from build123d import *

# Parameters (mm, degrees)
SKETCH1_R           = 2.1
BOSS_EXTRUDE1_DEPTH = 20
SKETCH2_W           = 74
SKETCH2_H           = 111
CUT_EXTRUDE1_DEPTH  = 18


with BuildPart() as part:
    # Sketch1 → Boss-Extrude1 (new body)
    with BuildSketch(Plane(origin=(0, 0, 0), x_dir=(1, 0, 0), z_dir=(0, 1, 0))):
        with BuildLine():
            Line((-55.8, 60), (55.8, 60))
            ThreePointArc((55.8, 60), (58.769848481, 58.769848481), (60, 55.8))
            Line((60, 55.8), (60, -55.8))
            ThreePointArc((60, -55.8), (58.769848481, -58.769848481), (55.8, -60))
            Line((55.8, -60), (-55.8, -60))
            ThreePointArc((-55.8, -60), (-58.769848481, -58.769848481), (-60, -55.8))
            Line((-60, -55.8), (-60, 55.8))
            ThreePointArc((-60, 55.8), (-58.769848481, 58.769848481), (-55.8, 60))
        make_face()
        with Locations(Location((50, 50, 0), (0, 0, 270))):
            Circle(SKETCH1_R, mode=Mode.SUBTRACT)
        with Locations(Location((-50, 50, 0), (0, 0, 90))):
            Circle(SKETCH1_R, mode=Mode.SUBTRACT)
        with Locations(Location((50, -50, 0), (0, 0, 90))):
            Circle(SKETCH1_R, mode=Mode.SUBTRACT)
        with Locations(Location((-50, -50, 0), (0, 0, 270))):
            Circle(SKETCH1_R, mode=Mode.SUBTRACT)
    extrude(amount=BOSS_EXTRUDE1_DEPTH)

    # Sketch2 → Cut-Extrude1 (cut)
    with BuildSketch(Plane(origin=(0, 20, 0), x_dir=(1, 0, 0), z_dir=(0, 1, 0))):
        Rectangle(SKETCH2_W, SKETCH2_H)
    extrude(amount=-CUT_EXTRUDE1_DEPTH, mode=Mode.SUBTRACT)


solid = part.part
Could you check a few things on this model? Use its own coordinates, in mm. A direction names the side the tool comes from. Round coordinates to 2 decimals unless told otherwise and drop trailing zeros. Write each loop counter-clockwise with the first axis right and the second up, starting at its lowest first coordinate (ties: lowest second). Pieces come first, ordered by that corner, then holes. Notation, with made-up numbers: (80.5, 82.5) -> (118.5, 82.5) arc R20 cw to (118.5, 87.5) -> close; hole circle Ø4 at (-18.5, 5.25). An arc over 180 degrees is marked (long way). Use a Markdown table: item, result.
1. We'd pull the mould along X, two halves only. Please class faces 3 (the face through (58.74, 9.86, -58.8)), 4 (the face through (-1, 2, -1)), 5 (the face through (-48.137, 9.86, -50.969)), 6 (the face through (-58.74, 9.86, 58.8)): +X half, -X half, draft (parallel to the pull), parting line (faces both ways), or undercut.
Answer key:
| item | result |
|---|---|
| face 3 | +X half |
| face 4 | undercut |
| face 5 | undercut |
| face 6 | -X half |
2. If we section it at B-B (y = 18): List the corners of the cut face in (x, z) for me.
Answer key:
| item | result |
|---|---|
| outline | (-60, -55.8) arc R4.2 ccw to (-55.8, -60) -> (55.8, -60) arc R4.2 ccw to (60, -55.8) -> (60, 55.8) arc R4.2 ccw to (55.8, 60) -> (-55.8, 60) arc R4.2 ccw to (-60, 55.8) -> close; hole circle Ø4.2 at (-50, -50); hole circle Ø4.2 at (-50, 50); hole (-37, -55.5) -> (37, -55.5) -> (37, 55.5) -> (-37, 55.5) -> close; hole circle Ø4.2 at (50, -50); hole circle Ø4.2 at (50, 50) |
3. Please list where these lines run through material, in increasing order: probe 1 along X at (y, z) = (8.75, -50); probe 2 along X at (y, z) = (2.5, -17); probe 3 along Z at (x, y) = (-18, 10.75).
Answer key:
| item | result |
|---|---|
| probe 1 | x = -60 to -52.1, -47.9 to -37, 37 to 47.9, 52.1 to 60 |
| probe 2 | x = -60 to -37, 37 to 60 |
| probe 3 | z = -60 to -55.5, 55.5 to 60 |
4. If we section it at A-A (z = -50): List the corners of the cut face in (x, y) for me.
Answer key:
| item | result |
|---|---|
| outline | (-60, 0) -> (-52.1, 0) -> (-52.1, 20) -> (-60, 20) -> close; (-47.9, 0) -> (47.9, 0) -> (47.9, 20) -> (37, 20) -> (37, 2) -> (-37, 2) -> (-37, 20) -> (-47.9, 20) -> close; (52.1, 0) -> (60, 0) -> (60, 20) -> (52.1, 20) -> close |
5. If we section it at D-D (z = 12): List the corners of the cut face in (x, y) for me.
Answer key:
| item | result |
|---|---|
| outline | (-60, 0) -> (60, 0) -> (60, 20) -> (37, 20) -> (37, 2) -> (-37, 2) -> (-37, 20) -> (-60, 20) -> close |
6. Which directions (+Z, -Z, +X, -X, +Y, -Y) give clear straight access to the entire face, cutting with the end or side of a thin tool? Please do faces 1 (the face through (-37, 11, 1)), 2 (the face through (-51.863, 9.86, 50.969)).
Answer key:
| item | result |
|---|---|
| face 1 | +Y |
| face 2 | +Y, -Y |
7. If we section it at C-C (x = -50): List the corners of the cut face in (y, z) for me, then the cut area to 3 significant figures.
Answer key:
| item | result |
|---|---|
| outline | (0, -60) -> (20, -60) -> (20, -52.1) -> (0, -52.1) -> close; (0, -47.9) -> (20, -47.9) -> (20, 47.9) -> (0, 47.9) -> close; (0, 52.1) -> (20, 52.1) -> (20, 60) -> (0, 60) -> close |
| area | 2,230 mm^2 |
